Geometry check sheet. Reference: the model listing, model coordinates, mm. A direction names the side the tool comes from. Coordinates: 2 decimals unless noted, no trailing zeros. Loops run counter-clockwise (first coordinate to the right, second up) from the corner with the lowest first, then second, coordinate; pieces in that order, holes last. Notation, with made-up numbers: M 54,34 L 98,34 A30 cw 98,61 Z; hole C 65,-13 d2. An arc over 180 degrees is marked long. Use CSV: the item, a comma, the result in double quotes.
```python
from build123d import *

# Parameters (mm, degrees)
F2_W            = 43
F2_H            = 20
F2_R            = 3.5
F3_DEPTH        = 6
F3_COPIES_COUNT = 3
F4_R            = 18.25
F5_DEPTH        = 30.001
F6_SIZE         = 1
F7_R            = 2


# Not quite as in the source:
# - a pattern or mirror of a feature is missing from the dataset's text; its kind, count and spacing are read off the source's solid


with BuildPart() as f1:
    # F0 (on Front) → F1 (revolve)
    with BuildSketch(Plane.XZ):
        Polygon((21.15, 30), (0, 30), (0, 0), (26.3, 0), (26.3, 20), (21.15, 20), align=None)
    revolve(axis=Axis((0, 0, 22.5), (0, 0, 1)))

    # F2 (on Front) → F3 (join, symmetric)
    with BuildSketch(Plane.XZ):
        with Locations((21.5, 10)):
            Rectangle(F2_W, F2_H)
        with Locations((35, 10)):
            Circle(F2_R, mode=Mode.SUBTRACT)
    f3 = extrude(amount=F3_DEPTH, both=True)

    # F3_copies: F3 ×3 about axis
    f3_copies_axis = Axis((0, 0, 0), (0, 0, 1))
    for i in range(1, F3_COPIES_COUNT):
        add(f3.rotate(f3_copies_axis, i * 360 / F3_COPIES_COUNT))

    # F4 (on Top) → F5 (cut, through all)
    with BuildSketch(Plane.XY):
        Circle(F4_R)
    extrude(amount=F5_DEPTH, mode=Mode.SUBTRACT)

    # F6
    f6_edges = [f1.edges().sort_by_distance(p)[0] for p in [
        (-21.15, 0, 30),
    ]]
    chamfer(f6_edges, length=F6_SIZE)

    # F7
    f7_edges = [f1.edges().sort_by_distance(p)[0] for p in [
        (25.606445, -6, 10),
        (25.606445, 6, 10),
        (-7.60707, 25.175831, 10),
        (-17.999375, 19.175831, 10),
        (-7.60707, -25.175831, 10),
        (-17.999375, -19.175831, 10),
    ]]
    fillet(f7_edges, radius=F7_R)


solid = f1.part
```
1. Section check C-C, the plane z = 10. Count the separate pieces of the cut face and the enclosed holes in it, plus the area to 3 significant figures.
The answers:
separate pieces,"4"
enclosed holes,"1"
area,"1,490 mm^2"
2. Section check A-A, the plane y = 0. Record the cut outline in (x, z), plus the area to 3 significant figures.
The answers:
outline,"M -26.3,0 L -18.25,0 L -18.25,30 L -20.15,30 L -21.15,29 L -21.15,20 L -26.3,20 Z; M 18.25,0 L 43,0 L 43,20 L 21.15,20 L 21.15,29 L 20.15,30 L 18.25,30 Z; hole C 35,10 d7"
area,"675 mm^2"
3. Section check D-D, the plane x = 0. Record the cut outline in (y, z), plus the area to 3 significant figures.
The answers:
outline,"M -26.3,0 L -18.25,0 L -18.25,30 L -20.15,30 L -21.15,29 L -21.15,20 L -26.3,20 Z; M 18.25,0 L 26.3,0 L 26.3,20 L 21.15,20 L 21.15,29 L 20.15,30 L 18.25,30 Z"
area,"379 mm^2"
4. Gauge pin test, flat ends, axial feed: P1, Ø4, axis at y = 7.5, z = 9.5, coming from the +X side; P2, Ø8, axis at x = 35, z = 10, coming from the +Y side; P3, Ø4, axis at x = 10.5, z = 13, coming from the +Y side; P4, Ø1.5, axis at y = 10.5, z = 19.5, coming from the -X side. Record the tip position at first contact, or that the pin passes through.
The answers:
P1,"x = 43"
P2,"y = 6"
P3,"y = 24.89"
P4,"x = -24.43"
5. Set-up check for faces 1 (the flat face through (-20.9, -24.2, 12.4)), 2 (the flat face through (31, 6, 10)), 3 (the flat face through (31, -6, 10)), 4 (the flat face through (-21.43, 37.28, 9.86)), 5 (the cylindrical face through (-18.235, -31.752, 6.895)): record each of +Z, -Z, +X, -X, +Y, -Y from which the full face is reachable in a straight line by a thin tool's end or side.
The answers:
face 1,"+Z, -Z, -X"
face 2,"+Z, -Z, +X, +Y"
face 3,"+Z, -Z, +X, -Y"
face 4,"+Z, -Z, -X, +Y"
face 5,"none"
6. Thickness scan on line 1 (Y direction, x = 0, z = 11.25); line 2 (X direction, y = 0, z = 15.5); line 3 (Y direction, x = -20, z = 1.5). Record the ranges inside material, lowest first. Write a range as [from, to].
The answers:
line 1,"[-26.3, -18.25], [18.25, 26.3]"
line 2,"[-26.3, -18.25], [18.25, 43]"
line 3,"[-38.11, -22.64], [-17.08, 17.08], [22.64, 38.11]"
7. Section check B-B, the plane x = 35. Record the cut outline in (y, z), plus the area to 3 significant figures.
The answers:
outline,"M -6,0 L 6,0 L 6,6.5 L -6,6.5 Z; M -6,13.5 L 6,13.5 L 6,20 L -6,20 Z"
area,"156 mm^2"
8. Release check for a two-part mould opening along Z. For faces 6 (the cylindrical face through (-4.58, -20.65, 24.56)), 7 (the flat face through (-5, -18, 0)), 8 (the cylindrical face through (32.2, 0.1, 7.9)) record: +Z half, -Z half, draft (parallel to the pull), parting line (faces both ways), or undercut.
The answers:
face 6,"draft"
face 7,"-Z half"
face 8,"undercut"
